Model file for the job. Use its own axes, mm. Round coordinates to 2 decimals unless told otherwise and drop trailing zeros. Order: outer loops, then holes, each group sorted by start corner. A loop starts at its lowest first (then second) coordinate and runs counter-clockwise, first axis right, second up. Notation, with made-up numbers: (3, 50) - (51, 50) arc R25 cw to (51, 69) - close; hole circle Ø10 at (69, -17). An arc over 180 degrees is marked (long way). Put each result on its own line as item: value. Start each with the question number.
Item 1: Saw through at C-C on z = 4.25. List the corners of the cut face in (x, y) (3 decimals).
Item 2: Saw through at D-D on x = 8.5. List the corners of the cut face in (y, z).
Item 3: Mould opens along X. For faces 1 (the face through (-3.27, 41.52, 3.13)), 2 (the face through (-9, 7, 6.35)), 3 (the face through (-34.325, -23.592, 3.131)) say: pulls with the +X half, pulls with the -X half, needs draft (parallel to the pull), parting line crosses it, or undercut.
Item 4: Saw through at A-A on y = -15.5. List the corners of the cut face in (x, z).
Item 5: Saw through at B-B on y = -5. List the corners of the cut face in (x, z), plus the area to 3 significant figures.
Item 6: Pin check, flat tips, straight feed: pin 1 Ø1.5 at (y, z) = (16, 3.5) entering from +X; pin 2 Ø5 at (x, y) = (-10, -2.5) entering from +Z. Stop position of each tip, or through.
Item 7: Probe probe 1 along X at (y, z) = (-13.5, 6); probe 2 along X at (y, z) = (27.94, 2); probe 3 along Y at (x, z) = (24.5, 4.75). List the from-to ranges inside material, lowest first.
```python
from build123d import *

# Parameters (mm, degrees)
F1_R     = 11.049
F2_DEPTH = 6.35


with BuildPart() as f2:
    # F1 (on face) → F2 (new body)
    with BuildSketch(Plane.XY):
        with BuildLine():
            ThreePointArc((13.9621660883, 27.472220007), (13.9654123098, 27.7061212363), (13.97, 27.94))
            ThreePointArc((13.97, 27.94), (-3.6157020601, 41.4339837933), (-12.0983748909, 20.955))
            ThreePointArc((-12.0983748909, 20.955), (-6.9849999951, 15.8416251063), (1.14e-08, 13.97))
            ThreePointArc((1.14e-08, 13.97), (9.7114883941, 17.8976948278), (13.9621660883, 27.472220007))
        make_face()
        with BuildLine():
            ThreePointArc((11.049, 27.94), (7.8128228253, 20.1271771747), (0, 16.891))
            ThreePointArc((0, 16.891), (-7.8128228253, 35.7528228253), (11.049, 27.94))
        make_face(mode=Mode.SUBTRACT)
        with BuildLine():
            ThreePointArc((1.14e-08, 13.97), (-6.9849999951, 15.8416251063), (-12.0983748909, 20.955))
            ThreePointArc((-12.0983748909, 20.955), (-19.3348001595, 7.9193573575), (-30.7727234686, -1.6445194791))
            ThreePointArc((-30.7727234686, -1.6445194791), (-20.3556031034, -0.5384516084), (-12.0983754336, -6.98499906))
            ThreePointArc((-12.0983754336, -6.98499906), (-12.0983746167, 6.9850004749), (1.14e-08, 13.97))
        make_face()
        with BuildLine():
            ThreePointArc((24.1967497817, 0), (16.525764733, 12.7847494365), (13.9621660883, 27.472220007))
            ThreePointArc((13.9621660883, 27.472220007), (9.7114883941, 17.8976948278), (1.14e-08, 13.97))
            ThreePointArc((1.14e-08, 13.97), (9.8782817372, 9.8782817292), (13.97, 0))
            ThreePointArc((13.97, 0), (13.4939839355, -3.6157015292), (12.0983754405, -6.984999048))
            ThreePointArc((12.0983754405, -6.984999048), (17.2117502577, -1.8716248343), (24.1967497817, 0))
        make_face()
        with BuildLine():
            ThreePointArc((13.97, 0), (9.8782817372, 9.8782817292), (1.14e-08, 13.97))
            ThreePointArc((1.14e-08, 13.97), (-12.0983746167, 6.9850004749), (-12.0983754336, -6.98499906))
            ThreePointArc((-12.0983754336, -6.98499906), (6.9e-09, -13.97), (12.0983754405, -6.984999048))
            ThreePointArc((12.0983754405, -6.984999048), (13.4939839355, -3.6157015292), (13.97, 0))
        make_face()
        with BuildLine():
            ThreePointArc((11.049, 0), (-7.8128228253, -7.8128228253), (0, 11.049))
            ThreePointArc((0, 11.049), (7.8128228253, 7.8128228253), (11.049, 0))
        make_face(mode=Mode.SUBTRACT)
        with BuildLine():
            ThreePointArc((-12.0983754336, -6.98499906), (-20.3556031034, -0.5384516084), (-30.7727234686, -1.6445194791))
            ThreePointArc((-30.7727234686, -1.6445194791), (-30.9769109858, -1.7586587835), (-31.1817497817, -1.8716251091))
            ThreePointArc((-31.1817497817, -1.8716251091), (-34.0750315149, -23.8482817332), (-12.0983748909, -20.955))
            ThreePointArc((-12.0983748909, -20.955), (-10.7027659885, -17.5857020601), (-10.2267497817, -13.97))
            ThreePointArc((-10.2267497817, -13.97), (-10.7027661289, -10.3542974157), (-12.0983754336, -6.98499906))
        make_face()
        with Locations((-24.1967497817, -13.97)):
            Circle(F1_R, mode=Mode.SUBTRACT)
        with BuildLine():
            ThreePointArc((38.1667497817, -13.97), (34.0750315149, -4.0917182668), (24.1967497817, 0))
            ThreePointArc((24.1967497817, 0), (17.2117502577, -1.8716248343), (12.0983754405, -6.984999048))
            ThreePointArc((12.0983754405, -6.984999048), (10.6441140583, -17.359242533), (16.8105573802, -25.8277005278))
            ThreePointArc((16.8105573802, -25.8277005278), (17.0114986761, -25.9474624527), (17.2117497817, -26.0683748909))
            ThreePointArc((17.2117497817, -26.0683748909), (31.1817497817, -26.0683748909), (38.1667497817, -13.97))
        make_face()
        with Locations((24.1967497817, -13.97)):
            Circle(F1_R, mode=Mode.SUBTRACT)
        with BuildLine():
            ThreePointArc((12.0983754405, -6.984999048), (6.9e-09, -13.97), (-12.0983754336, -6.98499906))
            ThreePointArc((-12.0983754336, -6.98499906), (-10.7027661289, -10.3542974157), (-10.2267497817, -13.97))
            ThreePointArc((-10.2267497817, -13.97), (-10.7027659885, -17.5857020601), (-12.0983748909, -20.955))
            ThreePointArc((-12.0983748909, -20.955), (2.8090354265, -20.704106794), (16.8105573802, -25.8277005278))
            ThreePointArc((16.8105573802, -25.8277005278), (10.6441140583, -17.359242533), (12.0983754405, -6.984999048))
        make_face()
    extrude(amount=F2_DEPTH)


solid = f2.part
```
Results found:
1. outline: (-31.182, -1.872) arc R13.97 ccw (long way) to (-12.098, -20.955) arc R40.786 cw to (16.811, -25.828) arc R40.786 cw to (17.212, -26.068) arc R13.97 ccw (long way) to (24.197, 0) arc R40.786 cw to (13.962, 27.472) arc R40.786 cw to (13.97, 27.94) arc R13.97 ccw (long way) to (-12.098, 20.955) arc R40.786 cw to start; hole circle Ø22.098 at (-24.197, -13.97); hole circle Ø22.098 at (0, 0); hole circle Ø22.098 at (0, 27.94); hole circle Ø22.098 at (24.197, -13.97)
2. outline: (-22.09, 0) - (-7.06, 0) - (-7.06, 6.35) - (-22.09, 6.35) - close; (7.06, 0) - (20.88, 0) - (20.88, 6.35) - (7.06, 6.35) - close; (35, 0) - (39.03, 0) - (39.03, 6.35) - (35, 6.35) - close
3. face 1: parting line crosses it
3. face 2: needs draft
3. face 3: undercut
4. outline: (-38.08, 0) - (-35.14, 0) - (-35.14, 6.35) - (-38.08, 6.35) - close; (-13.25, 0) - (13.25, 0) - (13.25, 6.35) - (-13.25, 6.35) - close; (35.14, 0) - (38.08, 0) - (38.08, 6.35) - (35.14, 6.35) - close
5. outline: (-34.91, 0) - (-30.65, 0) - (-30.65, 6.35) - (-34.91, 6.35) - close; (-17.75, 0) - (-9.85, 0) - (-9.85, 6.35) - (-17.75, 6.35) - close; (9.85, 0) - (17.75, 0) - (17.75, 6.35) - (9.85, 6.35) - close; (30.65, 0) - (34.91, 0) - (34.91, 6.35) - (30.65, 6.35) - close
5. area: 154 mm²
6. pin 1: stops at x = 15.7
6. pin 2: stops at z = 6.35
7. probe 1: x = -38.16 to -35.24, -13.16 to 13.16, 35.24 to 38.16
7. probe 2: x = -13.97 to -11.05, 11.05 to 13.97
7. probe 3: y = -27.94 to -25.01, -2.93 to 0
